```python
from build123d import *

# Parameters (mm, degrees)
SKETCH_1_W          = 50
SKETCH_1_H          = 35
EXTRUDE_1_DEPTH     = 6
SKETCH_2_W          = 12
SKETCH_2_H          = 30
EXTRUDE_2_DEPTH     = 23
SKETCH_7_W          = 13
SKETCH_7_H          = 15
EXTRUDE_3_DEPTH     = 7
SKETCH_8_W          = 13
SKETCH_8_H          = 9
SKETCH_8_W_2        = 2
SKETCH_8_H_2        = 5.5
CUT_EXTRUDE_4_DEPTH = 7
EXTRUDE_4_DEPTH     = 31
SKETCH_11_W         = 11
SKETCH_11_H         = 5
CUT_EXTRUDE_5_DEPTH = 21
SKETCH_12_W         = 31
SKETCH_12_H         = 25
EXTRUDE_5_DEPTH     = 4


with BuildPart() as part:
    # Эскиз1 → Бобышка-Вытянуть1 (new body)
    with BuildSketch(Plane.XY):
        Rectangle(SKETCH_1_W, SKETCH_1_H)
    extrude(amount=EXTRUDE_1_DEPTH)

    # Эскиз2 → Бобышка-Вытянуть2 (add)
    with BuildSketch(Plane.XY.offset(6)):
        with Locations((12, -2.5)):
            Rectangle(SKETCH_2_W, SKETCH_2_H)
    extrude(amount=EXTRUDE_2_DEPTH)

    # Эскиз7 → Бобышка-Вытянуть3 (add)
    with BuildSketch(Plane(origin=(18, 0, 0), x_dir=(0, 0, -1), z_dir=(1, 0, 0))):
        with Locations((-12.5, 0)):
            Rectangle(SKETCH_7_W, SKETCH_7_H)
    extrude(amount=EXTRUDE_3_DEPTH)

    # Эскиз8 → Вырез-Вытянуть4 (cut)
    with BuildSketch(Plane(origin=(25, 0, 0), x_dir=(0, 0, -1), z_dir=(1, 0, 0))):
        with Locations((-8.5, 0)):
            Rectangle(SKETCH_8_W, SKETCH_8_H)
        with Locations((-1, -7.25)):
            Rectangle(SKETCH_8_W_2, SKETCH_8_H_2)
        with Locations((-1, 0)):
            Rectangle(SKETCH_8_W_2, SKETCH_8_H)
        with Locations((-1, 7.25)):
            Rectangle(SKETCH_8_W_2, SKETCH_8_H_2)
    extrude(amount=-CUT_EXTRUDE_4_DEPTH, mode=Mode.SUBTRACT)

    # Эскиз9 → Бобышка-Вытянуть4 (add)
    with BuildSketch(Plane.ZY.offset(25)):
        Polygon((6, 17.5), (17, 12.5), (17, 7.5), (6, 7.5), align=None)
    extrude(amount=-EXTRUDE_4_DEPTH)

    # Эскиз11 → Вырез-Вытянуть5 (cut)
    with BuildSketch(Plane(origin=(6, 0, 0), x_dir=(0, 0, -1), z_dir=(1, 0, 0))):
        with Locations((-11.5, 15)):
            Rectangle(SKETCH_11_W, SKETCH_11_H)
    extrude(amount=-CUT_EXTRUDE_5_DEPTH, mode=Mode.SUBTRACT)

    # Эскиз12 → Бобышка-Вытянуть5 (add)
    with BuildSketch(Plane.XY.offset(6)):
        with Locations((-9.5, -5)):
            Rectangle(SKETCH_12_W, SKETCH_12_H)
    extrude(amount=EXTRUDE_5_DEPTH)


solid = part.part
```
The listing builds one solid part. Answer for the finished solid, in the listing's coordinates (mm). A direction names the side the tool comes from. Round coordinates to 2 decimals unless told otherwise and drop trailing zeros. Loops run counter-clockwise (first coordinate to the right, second up) from the corner with the lowest first, then second, coordinate; pieces in that order, holes last. Notation, with made-up numbers: (-40, 8) - (18, 8) arc R11 ccw to (18, 27) - close; hole circle Ø3 at (4, 9.5). An arc over 180 degrees is marked (long way). Return JSON: item names as keys, results as strings. Group by question number.
1. The part is cut by section B-B on y = -9. Determine the outline of the cut face in (x, z), then the cut area to 3 significant figures.
2. The mould has two halves that part along Y. Classify faces 6 (the flat face through (22, 4.5, 8)), 7 (the flat face through (21, 0, 19)), 8 (the flat face through (21, -7.5, 13)), 9 (the flat face through (21, 7.5, 13)): pulls with the +Y half, pulls with the -Y half, needs draft (parallel to the pull), parting line crosses it, or undercut.
3. The part is cut by section D-D on y = 14. Determine the outline of the cut face in (x, z).
4. The part is cut by section A-A on z = 17.75. Determine the outline of the cut face in (x, y).
5. Which of the six approach directions +Z, -Z, +X, -X, +Y, -Y give full straight-line access (tool end or side, diameter ignored) to faces 1 (the flat face through (-25, 0, 6)), 2 (the flat face through (-10, 7.5, 14)), 3 (the flat face through (5, 12.5, 15)), 4 (the flat face through (22, -10, 1)), 5 (the flat face through (-10, 10, 17))?
6. Consider probe 1 along Y at (x, z) = (21.5, 4.5); probe 2 along X at (y, z) = (-2, 4); probe 3 along Z at (x, y) = (-7, -15). Determine where each line is inside the solid, lowest interval first.
7. Each of these flat-tipped pins is pushed along its axis until it touches: P1, Ø5.5, axis at x = -16, z = 14, coming from the -Y side; P2, Ø2.5, axis at x = -12.5, y = 10, coming from the +Z side; P3, Ø7, axis at y = -1, z = 14.5, coming from the +X side; P4, Ø3, axis at y = 6.5, z = 21.5, coming from the -X side. Where does it stop, or does it pass through?
8. The part is cut by section C-C on x = -3. Determine the outline of the cut face in (y, z), then the cut area to 3 significant figures.
Resolved:
{
 "1": {"outline": "(-25, 0) - (18, 0) - (18, 2) - (25, 2) - (25, 6) - (18, 6) - (18, 29) - (6, 29) - (6, 10) - (-25, 10) - close", "area": "686 mm²"},
 "2": {"face 6": "undercut", "face 7": "needs draft", "face 8": "pulls with the -Y half", "face 9": "pulls with the +Y half"},
 "3": {"outline": "(-25, 0) - (25, 0) - (25, 6) - (-15, 6) - (-15, 13.7) - (-25, 13.7) - close"},
 "4": {"outline": "(6, -17.5) - (18, -17.5) - (18, -7.5) - (25, -7.5) - (25, 7.5) - (18, 7.5) - (18, 12.5) - (6, 12.5) - close"},
 "5": {"face 1": "+Z, -Z, -X, +Y, -Y", "face 2": "+Z, -X, -Y", "face 3": "+Z, +X, +Y", "face 4": "-Z, +X", "face 5": "+Z, -X, +Y, -Y"},
 "6": {"probe 1": "y = -17.5 to -4.5, 4.5 to 17.5", "probe 2": "x = -25 to 18", "probe 3": "z = 0 to 10"},
 "7": {"P1": "stops at y = 7.5", "P2": "stops at z = 17", "P3": "stops at x = 25", "P4": "stops at x = 6"},
 "8": {"outline": "(-17.5, 0) - (17.5, 0) - (17.5, 6) - (12.5, 6) - (12.5, 17) - (7.5, 17) - (7.5, 10) - (-17.5, 10) - close", "area": "365 mm²"}
}
